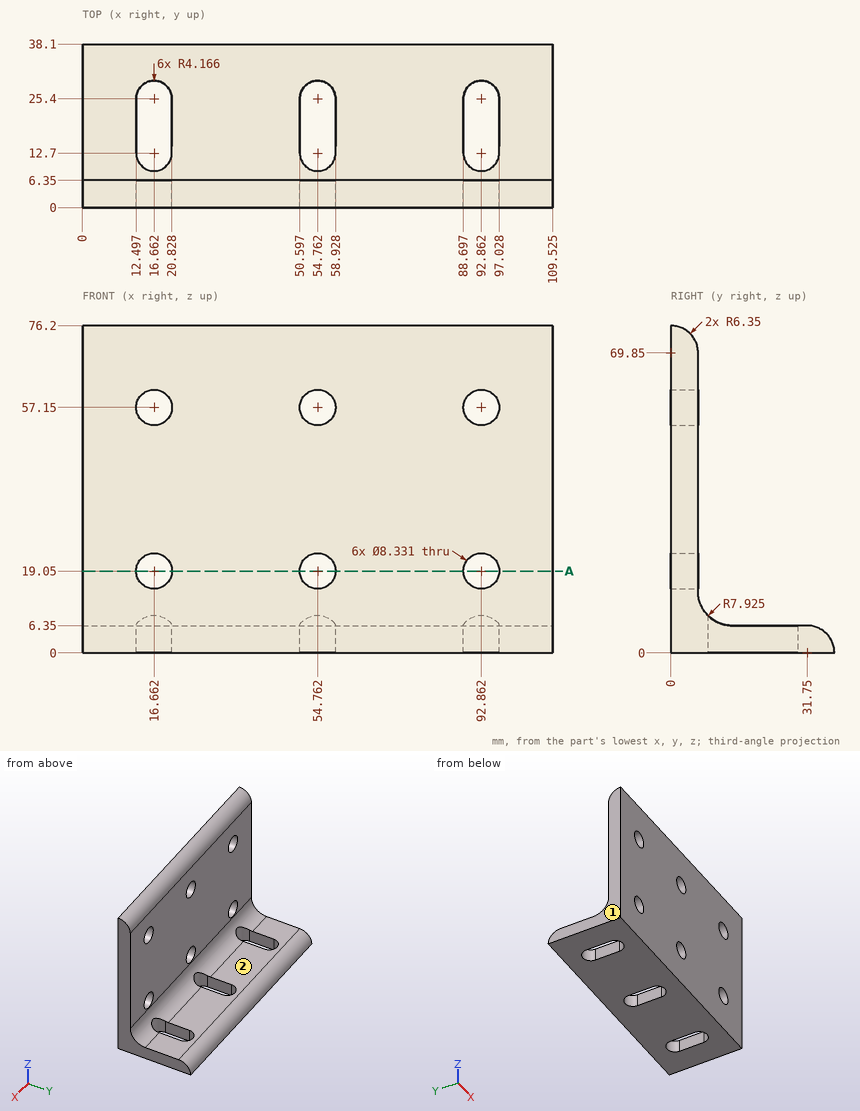
Geometry: see drawing. Coordinates: mm, zero at the bounding-box minimum. A direction names the side the tool comes from. Give positions to 0.01 mm unless a question says otherwise; leave off trailing zeros. Answer as a JSON object with one key per item and string values.
Q1. Access query for the marked faces 1 and 2. Directions: +Z, -Z, +X, -X, +Y, -Y. A direction counts if a zero-diameter tool reaches every point of the face in a straight line with its end or side. Return the directions, or none.
Geometry check:
{"face 1": "+Z, -Z, -X, +Y, -Y", "face 2": "+Z, +X, -X, +Y"}
Q2. Contact query for flat-ended pins moving along their axis: P1, Ø19, axis at x = 74.5, y = 25.5, coming from the +Z side; P2, Ø1, axis at x = 69, z = 24, coming from the +Y side; P3, Ø2, axis at x = 32, z = 12.5, coming from the +Y side. Output: stop coordinate, or through.
Geometry check:
{"P1": "stops at z = 6.35", "P2": "stops at y = 6.35", "P3": "stops at y = 6.85"}
Q3. Cut plane A-A, the plane z = 19.05. Count the separate pieces of the cut face and the enclosed holes in it, then the cut area to 3 significant figures.
Geometry check:
{"separate pieces": "4", "enclosed holes": "0", "area": "537 mm^2"}
Q4. Ray query, line 1 along X through (y, z) = (3.5, 57.15) (1 decimal); line 2 along Y through (x, z) = (13, 60). Return the intervals inside material, ascending.
Geometry check:
{"line 1": "x = 0 to 12.5, 20.8 to 50.6, 58.9 to 88.7, 97 to 109.5", "line 2": "y = 0 to 6.35"}
